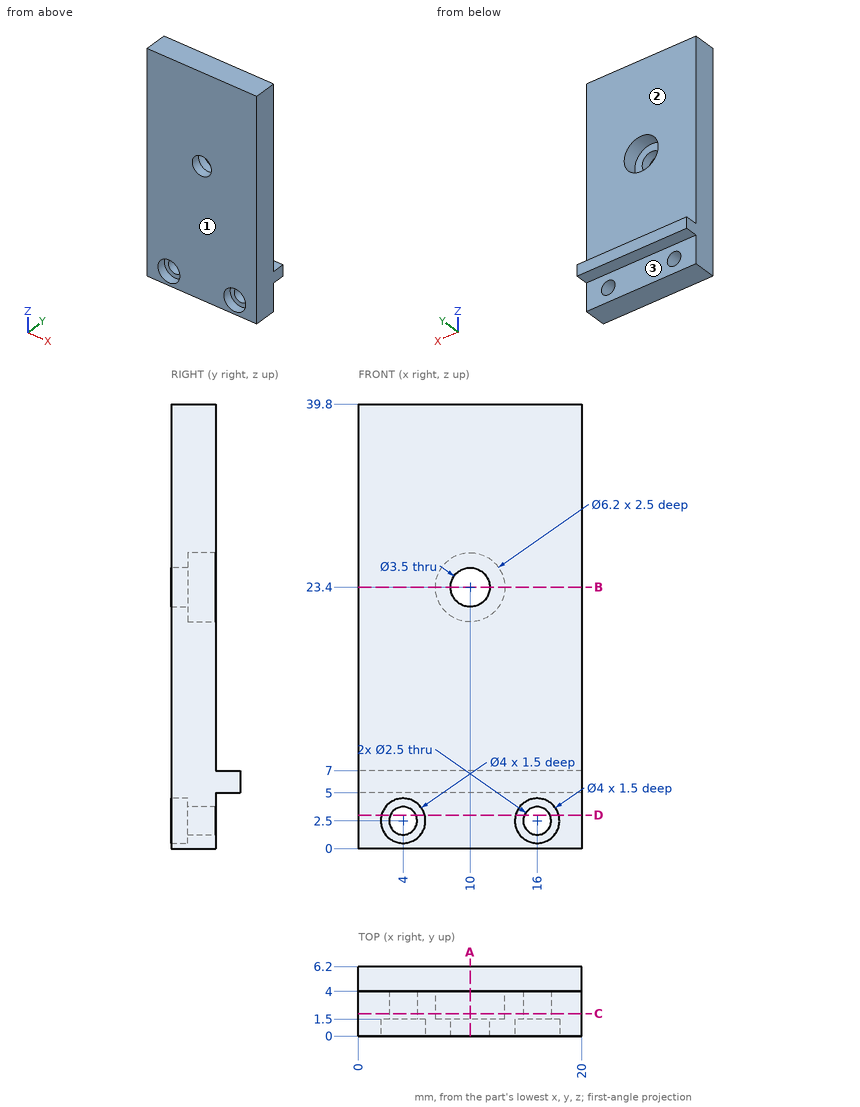
The figure shows three views and two pictorial views of one solid part (mm, origin at its lowest corner). Answer the questions. A direction names the side the tool comes from. Round coordinates to 2 decimals unless told otherwise and drop trailing zeros. Order: outer loops, then holes, each group sorted by start corner. A loop starts at its lowest first (then second) coordinate and runs counter-clockwise, first axis right, second up.
Q1. A cutting plane is placed at D-D, the plane z = 3. Determine the outline of the cut face in (x, y), then the cut area to 3 significant figures.
Solution:
outline: (0, 0) - (2.06, 0) - (2.06, 1.5) - (2.85, 1.5) - (2.85, 4) - (0, 4) - close; (5.15, 1.5) - (5.94, 1.5) - (5.94, 0) - (14.06, 0) - (14.06, 1.5) - (14.85, 1.5) - (14.85, 4) - (5.15, 4) - close; (17.15, 1.5) - (17.94, 1.5) - (17.94, 0) - (20, 0) - (20, 4) - (17.15, 4) - close
area: 56.9 mm2
Q2. A tool of negligible diameter and unlimited length cuts with its end or side. For the marked faces 1, 2 and 3, from which of +Z, -Z, +X, -X, +Y, -Y can it reach the whole face along a straight path? Write none if from no direction.
Solution:
face 1: +Z, -Z, +X, -X, -Y
face 2: +Z, +X, -X, +Y
face 3: -Z, +X, -X, +Y
Q3. Given pin 1 Ø2 at (x, y) = (2.5, 5.5) entering from -Z; pin 2 Ø1.5 at (x, z) = (9, 2) entering from +Y; pin 3 Ø0.7 at (x, y) = (5.5, 5) entering from +Z, each flat-ended and moving along its own axis, determine where each tip first touches the part or whether it passes through.
Solution:
pin 1: stops at z = 5
pin 2: stops at y = 4
pin 3: stops at z = 7
Q4. Find the intervals of material crossed by line 1 along X through (y, z) = (2.65, 2.5); line 2 along X through (y, z) = (0.7, 2.5); line 3 along X through (y, z) = (0.75, 23.4), in increasing order.
Solution:
line 1: x = 0 to 2.75, 5.25 to 14.75, 17.25 to 20
line 2: x = 0 to 2, 6 to 14, 18 to 20
line 3: x = 0 to 8.25, 11.75 to 20
Q5. A cutting plane is placed at A-A, the plane x = 10. Determine the outline of the cut face in (y, z), then the cut area to 3 significant figures.
Solution:
outline: (0, 0) - (4, 0) - (4, 5) - (6.2, 5) - (6.2, 7) - (4, 7) - (4, 20.3) - (1.5, 20.3) - (1.5, 21.65) - (0, 21.65) - close; (0, 25.15) - (1.5, 25.15) - (1.5, 26.5) - (4, 26.5) - (4, 39.8) - (0, 39.8) - close
area: 143 mm2
Q6. A cutting plane is placed at B-B, the plane z = 23.4. Determine the outline of the cut face in (x, y).
Solution:
outline: (0, 0) - (8.25, 0) - (8.25, 1.5) - (6.9, 1.5) - (6.9, 4) - (0, 4) - close; (11.75, 0) - (20, 0) - (20, 4) - (13.1, 4) - (13.1, 1.5) - (11.75, 1.5) - close
Q7. A cutting plane is placed at C-C, the plane y = 2. Determine the outline of the cut face in (x, z), then the cut area to 3 significant figures.
Solution:
outline: (0, 0) - (20, 0) - (20, 39.8) - (0, 39.8) - close; hole circle Ø2.5 at (4, 2.5); hole circle Ø6.2 at (10, 23.4); hole circle Ø2.5 at (16, 2.5)
area: 756 mm2
